Could you check a few things on this model? Use its own coordinates, in mm. Face numbers are marked on the shaded views. Give positions to 0.01 mm unless a question says otherwise; leave off trailing zeros. Loops run counter-clockwise (first coordinate to the right, second up) from the corner with the lowest first, then second, coordinate; pieces in that order, holes last. Notation, with made-up numbers: (57, 77.25) -> (76, 77.25) arc R22 cw to (76, 116.25) -> close; hole circle Ø10 at (7, 80). An arc over 180 degrees is marked (long way). Put each result on its own line as item: value.
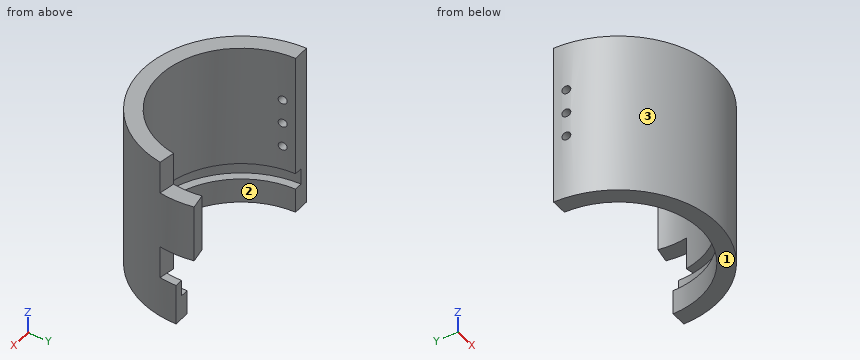
```python
from build123d import *

# Parameters (mm, degrees)
REVOLVE1_ANGLE     = 180
SKETCH2_W          = 10
SKETCH2_H          = 35
REVOLVE2_ANGLE     = 10
SKETCH3_W          = 10
SKETCH3_H          = 20
CUT_REVOLVE1_ANGLE = 10
CUT_EXTRUDE2_REACH = 142
SKETCH5_R          = 2.5


with BuildPart() as part:
    # Sketch1 → Revolve1 (revolve)
    with BuildSketch(Plane(origin=(0, 0, 0), x_dir=(1, 0, 0), z_dir=(0, 1, 0))):
        Polygon((-60, 19.117647059), (-60, -80.882352941), (-50, -80.882352941), (-50, -5.882352941), (-55, -5.882352941), (-55, 4.117647059), (-50, 4.117647059), (-50, 19.117647059), align=None)
    revolve(axis=Axis((0, 0, -69.117647059), (0, 0, 1)), revolution_arc=REVOLVE1_ANGLE)

    # Sketch2 → Revolve2 (revolve)
    with BuildSketch(Plane(origin=(0, 0, 0), x_dir=(1, 0, 0), z_dir=(0, 1, 0))):
        with Locations((55, -43.382352941)):
            Rectangle(SKETCH2_W, SKETCH2_H)
    revolve(axis=Axis((0, 0, -76.274402341), (0, 0, 1)), revolution_arc=REVOLVE2_ANGLE)

    # Sketch3 → Cut-Revolve1 (revolve, cut)
    with BuildSketch(Plane(origin=(0, 0, 0), x_dir=(1, 0, 0), z_dir=(0, 1, 0))):
        with Locations((55, -70.882352941)):
            Rectangle(SKETCH3_W, SKETCH3_H)
        with Locations((55, -15.882352941)):
            Rectangle(SKETCH3_W, SKETCH3_H)
    revolve(axis=Axis((0, 0, -76.834720656), (0, 0, -1)), revolution_arc=CUT_REVOLVE1_ANGLE, mode=Mode.SUBTRACT)

    # Sketch5 → Cut-Extrude2 (cut, up to next)
    with BuildSketch(Plane(origin=(-80, 0, 0), x_dir=(0, 0, -1), z_dir=(1, 0, 0)), mode=Mode.PRIVATE) as cut_extrude2_sk1:
        with Locations((-35.882352941, -7.5)):
            Circle(SKETCH5_R)
    cut_extrude2_tool1 = extrude(cut_extrude2_sk1.sketch, amount=CUT_EXTRUDE2_REACH, mode=Mode.PRIVATE) & part.part
    add(cut_extrude2_tool1.solids().sort_by_distance((-80, -7.5, 35.882353))[0], mode=Mode.SUBTRACT)
    # Sketch5 → Cut-Extrude2 (cut, up to next)
    with BuildSketch(Plane(origin=(-80, 0, 0), x_dir=(0, 0, -1), z_dir=(1, 0, 0)), mode=Mode.PRIVATE) as cut_extrude2_sk2:
        with Locations((-50.882352941, -7.5)):
            Circle(SKETCH5_R)
    cut_extrude2_tool2 = extrude(cut_extrude2_sk2.sketch, amount=CUT_EXTRUDE2_REACH, mode=Mode.PRIVATE) & part.part
    add(cut_extrude2_tool2.solids().sort_by_distance((-80, -7.5, 50.882353))[0], mode=Mode.SUBTRACT)
    # Sketch5 → Cut-Extrude2 (cut, up to next)
    with BuildSketch(Plane(origin=(-80, 0, 0), x_dir=(0, 0, -1), z_dir=(1, 0, 0)), mode=Mode.PRIVATE) as cut_extrude2_sk3:
        with Locations((-20.882352941, -7.5)):
            Circle(SKETCH5_R)
    cut_extrude2_tool3 = extrude(cut_extrude2_sk3.sketch, amount=CUT_EXTRUDE2_REACH, mode=Mode.PRIVATE) & part.part
    add(cut_extrude2_tool3.solids().sort_by_distance((-80, -7.5, 20.882353))[0], mode=Mode.SUBTRACT)


solid = part.part
```
1. If we section it at C-C (z = 17): List the corners of the cut face in (x, y) for me.
Recorded:
outline: (-60, 0) arc R60 ccw to (59.09, -10.42) -> (49.24, -8.68) arc R50 cw to (-50, 0) -> close
2. If we section it at D-D (y = -43): List the corners of the cut face in (x, z) for me, then the cut area to 3 significant figures.
Recorded:
outline: (-41.84, -19.12) -> (-25.51, -19.12) -> (-25.51, -4.12) -> (-34.29, -4.12) -> (-34.29, 5.88) -> (-25.51, 5.88) -> (-25.51, 80.88) -> (-41.84, 80.88) -> close; (25.51, -19.12) -> (41.84, -19.12) -> (41.84, 80.88) -> (25.51, 80.88) -> (25.51, 5.88) -> (34.29, 5.88) -> (34.29, -4.12) -> (25.51, -4.12) -> close
area: 3,090 mm^2
3. I need wall thicknesses on line 1 (Z direction, x = -55.75, y = -7.5); line 2 (Z direction, x = 16.5, y = -50.5); line 3 (Z direction, x = -57, y = -7). Which ranges of each line are inside material? Lowest first, please.
Recorded:
line 1: z = -19.12 to 18.38, 23.38 to 33.38, 38.38 to 48.38, 53.38 to 80.88
line 2: z = -19.12 to -4.12, 5.88 to 80.88
line 3: z = -19.12 to 18.43, 23.33 to 33.43, 38.33 to 48.43, 53.33 to 80.88
4. If we section it at B-B (x = 0): List the corners of the cut face in (y, z) for me.
Recorded:
outline: (-60, -19.12) -> (-50, -19.12) -> (-50, -4.12) -> (-55, -4.12) -> (-55, 5.88) -> (-50, 5.88) -> (-50, 80.88) -> (-60, 80.88) -> close
5. I'm going to push flat-ended pins straight in: pin 1 (1.5 mm diameter, centred on y = -37, z = 11.5, fed in from +X); pin 2 (6.5 mm diameter, centred on y = -7.5, z = 50.88, fed in from +X); pin 3 (6 mm diameter, centred on x = 33, z = 49.5, fed in from +Y); pin 4 (12 mm diameter, centred on x = 53.5, y = 3, fed in from -Z). Where does each tip first touch, or does it pass through?
Recorded:
pin 1: stops at x = 47.81
pin 2: stops at x = 59.85
pin 3: stops at y = -34.7
pin 4: stops at z = -19.12
6. If we section it at A-A (y = -25): List the corners of the cut face in (x, z) for me.
Recorded:
outline: (-54.54, -19.12) -> (-43.3, -19.12) -> (-43.3, -4.12) -> (-48.99, -4.12) -> (-48.99, 5.88) -> (-43.3, 5.88) -> (-43.3, 80.88) -> (-54.54, 80.88) -> close; (43.3, -19.12) -> (54.54, -19.12) -> (54.54, 80.88) -> (43.3, 80.88) -> (43.3, 5.88) -> (48.99, 5.88) -> (48.99, -4.12) -> (43.3, -4.12) -> close
7. Thinking about a two-plate mould opening in X: for the marked faces 1, 2 and 3, which applies, pulls with the +X half, pulls with the -X half, needs draft (parallel to the pull), parting line crosses it, or undercut?
Recorded:
face 1: needs draft
face 2: undercut
face 3: parting line crosses it
